from build123d import *

# Parameters (mm, degrees)
SKETCH026_W     = 20
SKETCH026_H     = 30
PAD008_DEPTH    = 40
SKETCH027_R     = 1.9
POCKET018_DEPTH = 20.001
SKETCH028_R     = 3
POCKET019_DEPTH = 3
SKETCH029_R     = 0.5
POCKET020_DEPTH = 0.5
SKETCH030_W     = 14.5
SKETCH030_H     = 14.5
POCKET021_DEPTH = 30
SKETCH031_W     = 14.5
SKETCH031_H     = 30
POCKET022_DEPTH = 5
SKETCH032_W     = 14.5
SKETCH032_H     = 6
POCKET023_DEPTH = 11.751
SKETCH033_W     = 2
SKETCH033_H     = 14
POCKET024_DEPTH = 18.25
SKETCH034_W     = 14.5
SKETCH034_H     = 10
POCKET025_DEPTH = 4


with BuildPart() as part:
    # Sketch026 → Pad008 (new body)
    with BuildSketch(Plane.XY):
        with Locations((-43, 0)):
            Rectangle(SKETCH026_W, SKETCH026_H)
    extrude(amount=PAD008_DEPTH)

    # Sketch027 (on Face4 of Pad008) → Pocket018 (cut, through all)
    with BuildSketch(Plane(origin=(-53, 0, 0), x_dir=(0, -1, 0), z_dir=(-1, 0, 0))):
        with Locations((-11, 36)):
            Circle(SKETCH027_R)
        with Locations((11, 20)):
            Circle(SKETCH027_R)
        with Locations((-11, 20)):
            Circle(SKETCH027_R)
        with Locations((-11, 4)):
            Circle(SKETCH027_R)
        with Locations((11, 4)):
            Circle(SKETCH027_R)
    extrude(amount=-POCKET018_DEPTH, mode=Mode.SUBTRACT)

    # Sketch028 (on Face2 of Pocket018) → Pocket019 (cut)
    with BuildSketch(Plane(origin=(-53, 0, 0), x_dir=(0, -1, 0), z_dir=(-1, 0, 0))):
        with Locations((-11, 36)):
            Circle(SKETCH028_R)
        with Locations((-11, 20)):
            Circle(SKETCH028_R)
        with Locations((-11, 4)):
            Circle(SKETCH028_R)
        with Locations((11, 4)):
            Circle(SKETCH028_R)
        with Locations((11, 20)):
            Circle(SKETCH028_R)
    extrude(amount=-POCKET019_DEPTH, mode=Mode.SUBTRACT)

    # Sketch029 (on Face5 of Pocket019) → Pocket020 (cut)
    with BuildSketch(Plane.XY.offset(40)):
        with Locations((-43, -4)):
            Circle(SKETCH029_R)
    extrude(amount=-POCKET020_DEPTH, mode=Mode.SUBTRACT)

    # Sketch030 (on Face5 of Pocket020) → Pocket021 (cut)
    with BuildSketch(Plane.XY.offset(40)):
        with Locations((-43, -4)):
            Rectangle(SKETCH030_W, SKETCH030_H)
    extrude(amount=-POCKET021_DEPTH, mode=Mode.SUBTRACT)

    # Sketch031 (on Face6 of Pocket021) → Pocket022 (cut)
    with BuildSketch(Plane.XZ.offset(15)):
        with Locations((-43, 25)):
            Rectangle(SKETCH031_W, SKETCH031_H)
    extrude(amount=-POCKET022_DEPTH, mode=Mode.SUBTRACT)

    # Sketch032 (on Face17 of Pocket022) → Pocket023 (cut, through all)
    with BuildSketch(Plane.XZ.offset(-3.25)):
        with Locations((-43, 13)):
            Rectangle(SKETCH032_W, SKETCH032_H)
    extrude(amount=-POCKET023_DEPTH, mode=Mode.SUBTRACT)

    # Sketch033 (on Face7 of Pocket023) → Pocket024 (cut)
    with BuildSketch(Plane.XZ.offset(15)):
        with Locations((-51.25, 19)):
            Rectangle(SKETCH033_W, SKETCH033_H)
        with Locations((-34.75, 19)):
            Rectangle(SKETCH033_W, SKETCH033_H)
    extrude(amount=-POCKET024_DEPTH, mode=Mode.SUBTRACT)

    # Sketch034 (on Face33 of Pocket024) → Pocket025 (cut)
    with BuildSketch(Plane.XZ.offset(-3.25)):
        with Locations((-43, 21)):
            Rectangle(SKETCH034_W, SKETCH034_H)
    extrude(amount=-POCKET025_DEPTH, mode=Mode.SUBTRACT)


solid = part.part
Can you work these out from the model? Positions are in its coordinate system, mm. A direction names the side the tool comes from. Round coordinates to 2 decimals unless told otherwise and drop trailing zeros. Write each loop counter-clockwise with the first axis right and the second up, starting at its lowest first coordinate (ties: lowest second). Pieces come first, ordered by that corner, then holes. Notation, with made-up numbers: (65.25, 57.5) -> (112.25, 57.5) arc R23 cw to (112.25, 90.5) -> close; hole circle Ø11 at (40.5, 42.5). An arc over 180 degrees is marked (long way). Use one line per item in the form item = value. Start each with the question number.
Q1. I'm going to push flat-ended pins straight in: P1, Ø1, axis at y = 11, z = 20.5, coming from the -X side; P2, Ø5, axis at x = -45, z = 18.5, coming from the -Y side; P3, Ø2, axis at x = -47.5, z = 34.5, coming from the -Y side; P4, Ø11.5, axis at x = -42.5, y = -5, coming from the +Z side. Where does each tip first touch, or does it pass through?
Q2. Which directions (+Z, -Z, +X, -X, +Y, -Y) give clear straight access to the entire face, cutting with the end or side of a thin tool? Please do faces 1 (the face through (-52.6, -8.6, 18.2)), 2 (the face through (-43, 7, 40)), 3 (the face through (-50.25, -6, 33)), 4 (the face through (-51, 3.25, 19)).
Q3. Imagine slicing it at C-C (z = 20). Please give me the cut outline in (x, y).
Q4. Imagine slicing it at B-B (y = 11). Count the separate pieces of the cut face and the enclosed holes in it, then the cut area to 3 significant figures.
Q5. If I drill on probe 1 along Z at (x, y) = (-38, 11); probe 2 along X at (y, z) = (-0.25, 13); probe 3 along X at (y, z) = (2.5, 27), over which ranges is the centre line in solid material (lowest first)? Write a range as [from, to].
Q6. We'd pull the mould along X, two halves only. Please class faces 5 (the face through (-33, 0, 20)), 6 (the face through (-35, -6, 26)), 7 (the face through (-33.38, -10.753, 21.884)): +X half, -X half, draft (parallel to the pull), parting line (faces both ways), or undercut.
Q7. Imagine slicing it at D-D (x = -38.5). Please give me the cut outline in (y, z).
Q8. Imagine slicing it at A-A (z = 36). Please give me the cut outline in (x, y), then the cut area to 3 significant figures.
Worked out:
q1.P1 = through
q1.P2 = 7.25
q1.P3 = 3.25
q1.P4 = 10
q2.face_1 = -X
q2.face_2 = +Z, +X, -X, +Y, -Y
q2.face_3 = +Z, -Y
q2.face_4 = -Y
q3.outline = (-53, -15) -> (-52.25, -15) -> (-52.25, -14) -> (-53, -14) -> close; (-53, -8) -> (-52.25, -8) -> (-52.25, 3.25) -> (-50.25, 3.25) -> (-50.25, 7.25) -> (-35.75, 7.25) -> (-35.75, 3.25) -> (-33.75, 3.25) -> (-33.75, -9.1) -> (-33, -9.1) -> (-33, 9.1) -> (-50, 9.1) -> (-50, 8) -> (-53, 8) -> close; (-53, 14) -> (-50, 14) -> (-50, 12.9) -> (-33, 12.9) -> (-33, 15) -> (-53, 15) -> close; (-33.75, -15) -> (-33, -15) -> (-33, -12.9) -> (-33.75, -12.9) -> close
q4.separate_pieces = 4
q4.enclosed_holes = 1
q4.area = 465 mm^2
q5.probe_1 = [0, 2.1], [5.9, 10], [16, 18.1], [21.9, 34.1], [37.9, 40]
q5.probe_2 = [-53, -52.25], [-33.75, -33]
q5.probe_3 = [-53, -50.25], [-35.75, -33]
q6.face_5 = +X half
q6.face_6 = undercut
q6.face_7 = draft
q7.outline = (-15, 0) -> (15, 0) -> (15, 10) -> (-15, 10) -> close; (3.25, 26) -> (7.25, 26) -> (7.25, 16) -> (15, 16) -> (15, 40) -> (3.25, 40) -> close; hole circle Ø3.8 at (-11, 4); hole circle Ø3.8 at (11, 4); hole circle Ø3.8 at (11, 20); hole circle Ø3.8 at (11, 36)
q8.outline = (-53, -15) -> (-50.25, -15) -> (-50.25, 3.25) -> (-35.75, 3.25) -> (-35.75, -15) -> (-33, -15) -> (-33, 9.1) -> (-50, 9.1) -> (-50, 8) -> (-53, 8) -> close; (-53, 14) -> (-50, 14) -> (-50, 12.9) -> (-33, 12.9) -> (-33, 15) -> (-53, 15) -> close
q8.area = 253 mm^2
